Autodesk Inventor part; units mm, degrees
ref_plane "YZ Plane" through (0, 0, 0) normal (1, 0, 0) x (0, 1, 0)
ref_plane "XZ Plane" through (0, 0, 0) normal (0, 1, 0) x (-1, 0, 0)
ref_plane "XY Plane" through (0, 0, 0) normal (0, 0, 1) x (1, 0, 0)
sketch "Sketch1" plane through (0, 0, 0) normal (0, 0, 1) x (1, 0, 0)
  line L0 (0, 0) -> (0, 177.8)
  line L1 (0, 0) -> (53.8815, 0) construction
  line L2 (0, 177.8) -> (71.6046, 151.7381)
  line L3 (0, 177.8) -> (76.2, 177.8) construction
  line L4 (71.6046, 151.7381) -> (0, 0)
  dimension "d0" = 177.8
  dimension "d19" = 76.2
  dimension "d20" = 20
extrude "Extrusion1" add sketch "Sketch1" along normal blind 6.35
fillet "Fillet1" radius 6.35 2 edges at (0, 177.8, 3.175) (0, 0, 3.175)
fillet "Fillet4" radius 6.35 1 edges at (71.6046, 151.7381, 3.175)
sketch "Sketch3" plane through (0, 0, 6.35) normal (0, 0, 1) x (1, 0, 0)
  circle A0 centre (3.175, 58.1807) radius 1.524
  circle A1 centre (3.175, 89.9307) radius 1.524
  line L0 (0, 168.7313) -> (0, 28.3357)
  point P0 (0, 0)
  dimension "d22" = 3.048
  dimension "d23" = 3.048
  dimension "d24" = 3.175
  dimension "d25" = 3.175
  dimension "d26" = 29.845
  dimension "d27" = 31.75
extrude "Extrusion3" cut sketch "Sketch3" against normal through all
sketch "Sketch4" plane through (0, 0, 6.35) normal (0, 0, 1) x (1, 0, 0)
  circle A0 centre (3.175, 58.1807) radius 1.524
  circle A1 centre (3.175, 58.1807) radius 2.921
  circle A2 centre (3.175, 89.9307) radius 1.524
  circle A3 centre (3.175, 89.9307) radius 2.921
  point P0 (0, 0)
  dimension "d30" = 5.842
  dimension "d31" = 5.842
extrude "Extrusion4" cut sketch "Sketch4" against normal blind 3.556
sketch "Sketch5" plane through (0, 0, 6.35) normal (0, 0, 1) x (1, 0, 0)
  circle A0 centre (60.795, 143.1007) radius 3.175
  point P0 (0, 0)
  point P1 (8.5218, 174.6983)
  dimension "d34" = 6.35
  dimension "d35" = 52.2732
  dimension "d36" = 31.5976
extrude "Extrusion5" cut sketch "Sketch5" against normal through all
sketch "Sketch6" plane through (0, 0, 6.35) normal (0, 0, 1) x (1, 0, 0)
  line L0 (0, 168.7313) -> (0, 28.3357)
  arc A0 (8.5218, 174.6983) -> (0, 168.7313) centre (6.35, 168.7313) ccw
  point P0 (0, 0)
  point P1 (10.0076, 166.8263)
  point P2 (10.0076, 31.8263)
  dimension "d39" = 10.0076
  dimension "d40" = 1.905
  dimension "d41" = 136.905
  dimension "d42" = 0
hole "Hole1" at (10.0076, 31.8263, 6.35) at (10.0076, 166.8263, 6.35) direction (0, 0, -1) diameter 3 end through all
sketch "Sketch7" plane through (0, 0, 6.35) normal (0, 0, 1) x (1, 0, 0)
  line L0 (65.0627, 154.1191) -> (8.5218, 174.6983)
  line L1 (12.0927, 25.6258) -> (68.6335, 145.4421)
  circle A0 centre (48.6603, 139.0056) radius 1.5875
  circle A1 centre (54.0562, 154.0707) radius 1.5875
  point P0 (0, 0)
  dimension "d52" = 3.81
  dimension "d53" = 19.812
  dimension "d54" = 15.3162
  dimension "d55" = 16.8656
  dimension "d56" = 3.175
  dimension "d57" = 3.175
extrude "Extrusion6" cut sketch "Sketch7" against normal through all
equation "\"d22\" = d23"
properties part number "Triangle axle slide connector"
Check sheet for the modelled part. Datum: model origin and axes. Units: mm. A direction names the side the tool comes from. Coordinates: 2 decimals unless noted, no trailing zeros. Loops run counter-clockwise (first coordinate to the right, second up) from the corner with the lowest first, then second, coordinate; pieces in that order, holes last.
1) Material ranges on probe 1 along X at (y, z) = (153.5, 0.5); probe 2 along Y at (x, z) = (3, 5); probe 3 along X at (y, z) = (134, 4), recorded low to high.
2) Access from +Z, -Z, +X, -X, +Y, -Y to the whole of each face (thin tool, end or side, straight path). Record for faces 1 (the face through (0, 98, 3)), 2 (the face through (4.4, 88.7, 2.794)).
3) Sectioned sample at A-A (z = 1.25). Count the separate pieces of the cut face and the enclosed holes in it, and give its area (3 significant figures).
4) Sectioned sample at B-B (x = 59). Record the boundary of the cut face in (y, z), and give its area (3 significant figures).
5) Release check for a two-part mould opening along Y. For faces 3 (the face through (54.91, 155.41, 3.22)), 4 (the face through (26, 117, 0)), 5 (the face through (4.845, 22.167, 3.219)) record: released by +Y, released by -Y, zero draft, split by the parting line, or undercut.
6) Gauge pin test, flat ends, axial feed: pin 1 (4 mm diameter, centred on x = 60.8, y = 143.1, fed in from -Z); pin 2 (2 mm diameter, centred on x = 59.5, z = 3.5, fed in from -Y); pin 3 (1.8 mm diameter, centred on x = 4, y = 59, fed in from +Z). Record the tip position at first contact, or that the pin passes through.
7) Sectioned sample at C-C (y = 73). Record the boundary of the cut face in (x, z).
8) Sectioned sample at D-D (x = 14.5). Record the boundary of the cut face in (y, z).
Check sheet entries:
1. probe 1: x = 0 to 52.57, 55.54 to 66.31
1. probe 2: y = 22.94 to 55.26, 61.1 to 87.01, 92.85 to 174.13
1. probe 3: x = 0 to 63.23
2. face 1: +Z, -Z, -X, +Y, -Y
2. face 2: +Z
3. separate pieces: 1
3. enclosed holes: 7
3. area: 6,130 mm2
4. outline: (125.03, 0) - (140.48, 0) - (140.48, 6.35) - (125.03, 6.35) - close; (145.72, 0) - (156.33, 0) - (156.33, 6.35) - (145.72, 6.35) - close
4. area: 165 mm2
5. face 3: undercut
5. face 4: zero draft
5. face 5: released by -Y
6. pin 1: passes through
6. pin 2: stops at y = 123.97
6. pin 3: stops at z = 2.79
7. outline: (0, 0) - (34.45, 0) - (34.45, 6.35) - (0, 6.35) - close
8. outline: (30.73, 0) - (172.52, 0) - (172.52, 6.35) - (30.73, 6.35) - close
